```python
from build123d import *

# Parameters (mm, degrees)
SKETCH2_R               = 2.5
CUT_EXTRUDE1_DEPTH      = 38.389838192
CUT_EXTRUDE2_DEPTH      = 27.944387171
CUT_EXTRUDE2_DEPTH_BACK = 27.944387171
SKETCH3_R               = 1.55
SKETCH4_W               = 8
SKETCH4_H               = 5
CUT_EXTRUDE3_DEPTH      = 0.75
SKETCH5_R               = 2.5
CUT_EXTRUDE4_DEPTH      = 2
CHAMFER1_SIZE           = 0.25


with BuildPart() as part:
    # Sketch1 → Revolve1 (revolve)
    with BuildSketch(Plane.XY, mode=Mode.PRIVATE) as revolve1_sk:
        with BuildLine():
            Line((34, 0), (34, 4))
            Line((34, 4), (31.25, 4))
            ThreePointArc((31.25, 4), (30.5, 3.25), (29.75, 4))
            Line((29.75, 4), (22, 4))
            Line((22, 4), (22, 11))
            Line((22, 11), (20, 11))
            Line((20, 11), (20, 4))
            Line((20, 4), (0, 4))
            Line((0, 4), (0, 0))
            Line((0, 0), (34, 0))
        make_face()
    revolve(revolve1_sk.sketch.rotate(Axis((0, 0, 0), (1, 0, 0)), 90), axis=Axis((0, 0, 0), (1, 0, 0)))

    # Sketch2 → Cut-Extrude1 (cut, through all)
    with BuildSketch(Plane(origin=(34, 0, 0), x_dir=(0, 0, -1), z_dir=(1, 0, 0))):
        Circle(SKETCH2_R)
    extrude(amount=-CUT_EXTRUDE1_DEPTH, mode=Mode.SUBTRACT)

    # Sketch3 → Cut-Extrude2 (cut, two sides: drawn at the far end of the back side and taken through both)
    with BuildSketch(Plane(origin=(22, 0, 0), x_dir=(0, 0, -1), z_dir=(1, 0, 0)).offset(-CUT_EXTRUDE2_DEPTH_BACK)):
        with Locations((4.949747468, 4.949747468)):
            Circle(SKETCH3_R)
        with Locations((4.949747468, -4.949747468)):
            Circle(SKETCH3_R)
        with Locations((-4.949747468, -4.949747468)):
            Circle(SKETCH3_R)
        with Locations((-4.949747468, 4.949747468)):
            Circle(SKETCH3_R)
    extrude(amount=CUT_EXTRUDE2_DEPTH + CUT_EXTRUDE2_DEPTH_BACK, mode=Mode.SUBTRACT)

    # Sketch4 → Cut-Extrude3 (cut)
    with BuildSketch(Plane(origin=(0, 4, 0), x_dir=(1, 0, 0), z_dir=(0, 1, 0))):
        with Locations((7.5, 0)):
            Rectangle(SKETCH4_W, SKETCH4_H)
    extrude(amount=-CUT_EXTRUDE3_DEPTH, mode=Mode.SUBTRACT)

    # Sketch5 → Cut-Extrude4 (cut)
    with BuildSketch(Plane(origin=(0, 3.25, 0), x_dir=(1, 0, 0), z_dir=(0, 1, 0))):
        with Locations(Location((7.5, 0, 0), (0, 0, 248.865707785))):
            Circle(SKETCH5_R)
    extrude(amount=-CUT_EXTRUDE4_DEPTH, mode=Mode.SUBTRACT)

    # Chamfer1
    chamfer1_edges = [part.edges().sort_by_distance(p)[0] for p in [
        (22, 0, -11),
        (20, 0, -11),
        (0, 0, -4),
        (34, 0, -4),
    ]]
    chamfer(chamfer1_edges, length=CHAMFER1_SIZE)


solid = part.part
```
For this review, take the finished solid that the model builds, in its own axes (mm). A direction names the side the tool comes from. Coordinates: 2 decimals unless noted, no trailing zeros. Write each loop counter-clockwise with the first axis right and the second up, starting at its lowest first coordinate (ties: lowest second). Pieces come first, ordered by that corner, then holes. Notation, with made-up numbers: (29, 72.5) - (39, 72.5) arc R5 ccw to (39, 79.5) - close; hole circle Ø10 at (15.5, -8.5). An arc over 180 degrees is marked (long way). Answer in a Markdown table with one row per item. Add a question column.
Q1. We need section C-C, the plane x = 13. State the section outline as (y, z) points, and give its area (3 significant figures).
Q2. We need section B-B, the plane z = 0. Count the separate pieces of the cut face and the enclosed holes in it, and give its area (3 significant figures).
Q3. For P1, Ø2, axis at y = -4.5, z = -8.5, coming from the -X side; P2, Ø3.5, axis at x = 10.5, z = 0.5, coming from the +Y side; P3, Ø2.5, axis at x = 5.5, z = 1, coming from the +Y side, all flat-tipped, find the tip position at first contact; note any pin that passes through.
Q4. Draft analysis for pull direction Z (two halves, no side actions). For faces 1 (the cylindrical face through (21, 5, -3.4)), 2 (the flat face through (22, 0, -5)), 3 (the cylindrical face through (20.99, 10.74, -2.38)), state which applies: +Z half, -Z half, draft (parallel to the pull), parting line (faces both ways), or undercut.
Q5. We need section A-A, the plane y = 0. State the section outline as (x, z) points, and give its area (3 significant figures).
Q6. Tool access review of faces 4 (the flat face through (20, 0, 5)), 5 (the cylindrical face through (9, 2, -2)), 6 (the cylindrical face through (21, -4.9, -3.4)), 7 (the flat face through (4, 3.25, 0)), 8 (the cylindrical face through (25.821, 3.905, -0.867)): name each direction out of +Z, -Z, +X, -X, +Y, -Y from which nothing blocks a thin tool from reaching the whole face with its end or side.
Q7. For probe 1 along Y at (x, z) = (21.5, 0); probe 2 along X at (y, z) = (2.75, -6.25); probe 3 along Y at (x, z) = (16, -1.25), list the stretches that pass through material, from the lowest coordinate up.
Answer list:
| question | item | result |
|---|---|---|
| 1 | outline | circle Ø8 at (0, 0); hole circle Ø5 at (0, 0) |
| 1 | area | 30.6 mm2 |
| 2 | separate pieces | 3 |
| 2 | enclosed holes | 0 |
| 2 | area | 118 mm2 |
| 3 | P1 | stops at x = 20 |
| 3 | P2 | stops at y = 4 |
| 3 | P3 | stops at y = 3.25 |
| 4 | face 1 | undercut |
| 4 | face 2 | draft |
| 4 | face 3 | parting line |
| 5 | outline | (0, -3.75) - (0.25, -4) - (20, -4) - (20, -10.75) - (20.25, -11) - (21.75, -11) - (22, -10.75) - (22, -4) - (29.75, -4) arc R0.75 cw to (31.25, -4) - (33.75, -4) - (34, -3.75) - (34, -2.5) - (0, -2.5) - close; (0, 2.5) - (34, 2.5) - (34, 3.75) - (33.75, 4) - (31.25, 4) arc R0.75 cw to (29.75, 4) - (22, 4) - (22, 10.75) - (21.75, 11) - (20.25, 11) - (20, 10.75) - (20, 4) - (0.25, 4) - (0, 3.75) - close |
| 5 | area | 128 mm2 |
| 6 | face 4 | -X |
| 6 | face 5 | +Y |
| 6 | face 6 | +X, -X |
| 6 | face 7 | +Z, -Z, +Y |
| 6 | face 8 | +X |
| 7 | probe 1 | y = -11 to -2.5, 2.5 to 11 |
| 7 | probe 2 | x = 20 to 22 |
| 7 | probe 3 | y = -3.8 to -2.17, 2.17 to 3.8 |
